Autodesk Inventor part; units mm, degrees
ref_plane "YZ Plane" through (0, 0, 0) normal (1, 0, 0) x (0, 1, 0)
ref_plane "XZ Plane" through (0, 0, 0) normal (0, 1, 0) x (-1, 0, 0)
ref_plane "XY Plane" through (0, 0, 0) normal (0, 0, 1) x (1, 0, 0)
sketch "Sketch_1" plane through (0, 0, 0) normal (0, 0, 1) x (1, 0, 0)
  line L0 (31.75, 0) -> (0, 0)
  line L1 (0, 6.985) -> (0.635, 6.35)
  line L2 (0.635, 6.35) -> (31.115, 6.35)
  line L3 (31.115, 6.35) -> (31.75, 6.985)
  line L4 (31.75, 6.985) -> (31.75, 10.3505)
  arc A0 (31.75, 10.3505) -> (30.988, 11.1125) centre (30.988, 10.3505) ccw
  line L5 (30.988, 11.1125) -> (28.1559, 11.1125)
  line L6 (28.1559, 11.1125) -> (28.1559, 10.4267)
  line L7 (28.1559, 10.4267) -> (26.9875, 10.4267)
  line L8 (26.9875, 10.4267) -> (26.9875, 11.1125)
  line L9 (26.9875, 11.1125) -> (4.7625, 11.1125)
  line L10 (4.7625, 11.1125) -> (4.7625, 10.4267)
  line L11 (4.7625, 10.4267) -> (3.5941, 10.4267)
  line L12 (3.5941, 10.4267) -> (3.5941, 11.1125)
  line L13 (3.5941, 11.1125) -> (0.762, 11.1125)
  arc A1 (0.762, 11.1125) -> (0, 10.3505) centre (0.762, 10.3505) ccw
  line L14 (0, 10.3505) -> (0, 6.985)
revolve "Revolution1" add sketch "Sketch_1" angle 360 about axis through (31.75, 0, 0) along (1, 0, 0)
properties part number "U-LMU0 50"
Can you work these out from the model? Positions are in its coordinate system, mm. A direction names the side the tool comes from. Give positions to 0.01 mm unless a question says otherwise; leave off trailing zeros. One line per question, with ' | ' between items. Start each with the question number.
Q1. If I drill on line 1 (Z direction, x = 19.5, y = 0); line 2 (Y direction, x = 18, z = 2.5); line 3 (X direction, y = 7.25, z = -8), over which ranges is the centre line in solid material (lowest first)? Write a range as from..to.
Q2. If we mould it in two halves opening along X, with no side actions, what happens to faces 1 (the cylindrical face through (27.56, -2.26, 10.18)), 2 (the cylindrical face through (29.55, 10.6, -3.34)), 3 (the flat face through (31.75, 7, -2))? For each: +X half, -X half, draft (parallel to the pull), parting line (faces both ways), or undercut.
Q3. For pin 1 Ø2 at (x, z) = (23, 2) entering from -Y; pin 2 Ø8 at (x, z) = (18.5, 5.5) entering from -Y; pin 3 Ø2 at (x, z) = (22.5, -8.5) entering from +Y, each with a flat end and sliding along its axis, tell me the tip position at first contact or that it passes through.
Q4. For faces 4 (the cylindrical face through (2.16, 10.6, -3.34)), 5 (the flat face through (4.762, 7, -8)), which set-ups out of +Z, -Z, +X, -X, +Y, -Y let a thin tool reach every point of the face, with its end or its side?
Computed:
1) line 1: z = -11.11..-6.35, 6.35..11.11 | line 2: y = -10.83..-5.84, 5.84..10.83 | line 3: x = 0.14..3.59, 4.76..26.99, 28.16..31.61
2) face 1: undercut | face 2: draft | face 3: +X half
3) pin 1: stops at y = -11.07 | pin 2: stops at y = -11.01 | pin 3: stops at y = 8.2
4) face 4: +X, -X | face 5: none
